Verification items for the finished model (mm, model axes). Face numbers are marked on the shaded views. A direction names the side the tool comes from. Give positions to 0.01 mm unless a question says otherwise; leave off trailing zeros. Write each loop counter-clockwise with the first axis right and the second up, starting at its lowest first coordinate (ties: lowest second). Pieces come first, ordered by that corner, then holes. Notation, with made-up numbers: (-11, 75.5) -> (18, 75.5) arc R11 cw to (18, 92.5) -> close; hole circle Ø3 at (8.25, -40). An arc over 180 degrees is marked (long way). Write item = value, one per line.
from build123d import *

# Parameters (mm, degrees)
F0_W      = 31.75
F0_H      = 31.75
F1_DEPTH  = 3.175
F3_D      = 2.54
F3_DEPTH  = 1.27
F3_TIP    = 0.7630929862
F4_W      = 31.75
F4_H      = 5.1026814207
F5_DEPTH  = 38.1
F6_W      = 21.6686837375
F6_H      = 5.1026814207
F7_DEPTH  = 19.05
F8_W      = 11.3971428946
F8_H      = 5.1026814207
F9_DEPTH  = 12.7
F10_W     = 5.5938977748
F10_H     = 5.1191067934
F11_DEPTH = 5.08
F12_SIZE  = 2.54
F14_ANGLE = -90
F15_R     = 1.5379719929
F16_DEPTH = 1.905


with BuildPart() as f1:
    # F0 (on Top) → F1 (new body)
    with BuildSketch(Plane.XY):
        Rectangle(F0_W, F0_H)
    extrude(amount=F1_DEPTH)

    # F3
    with Locations(Plane.XY.offset(3.175)):
        with Locations((-2.5495558511, 2.3657830898)):
            Hole(F3_D / 2, depth=F3_DEPTH)
            with Locations((0, 0, -(F3_DEPTH + F3_TIP / 2))):  # 118° drill point
                Cone(0, F3_D / 2, F3_TIP, mode=Mode.SUBTRACT)

    # F4 (on face) → F5 (join)
    with BuildSketch(Plane.XY.offset(3.175)):
        with Locations((0, 13.3236592896)):
            Rectangle(F4_W, F4_H)
    extrude(amount=F5_DEPTH)

    # F6 (on face) → F7 (join)
    with BuildSketch(Plane.XY.offset(41.275)):
        with Locations((0, 13.3236592896)):
            Rectangle(F6_W, F6_H)
    extrude(amount=F7_DEPTH)

    # F8 (on face) → F9 (join)
    with BuildSketch(Plane.XY.offset(60.325)):
        with Locations((0, 13.3236592896)):
            Rectangle(F8_W, F8_H)
    extrude(amount=F9_DEPTH)

    # F10 (on face) → F11 (join)
    with BuildSketch(Plane.XZ.offset(-10.7723185793)):
        with Locations((0, 70.4654466033)):
            Rectangle(F10_W, F10_H)
    extrude(amount=F11_DEPTH)

    # F12
    f12_edges = [f1.edges().sort_by_distance(p)[0] for p in [
        (0, 5.692319, 67.905893),
    ]]
    chamfer(f12_edges, length=F12_SIZE)


with BuildPart() as f1_1:
    # F14: moved
    add(f1.part.rotate(Axis((0, 15.8751159906, 0), (1, 0, 0)), F14_ANGLE))

    # F15 (on face) → F16 (join)
    with BuildSketch(Plane(origin=(0, 38.0691058929, -38.0691058929), x_dir=(1, 0, 0), z_dir=(0, -0.7071067812, 0.7071067812))):
        with Locations((0, 66.584341228)):
            Circle(F15_R)
    extrude(amount=F16_DEPTH)


solid = f1_1.part
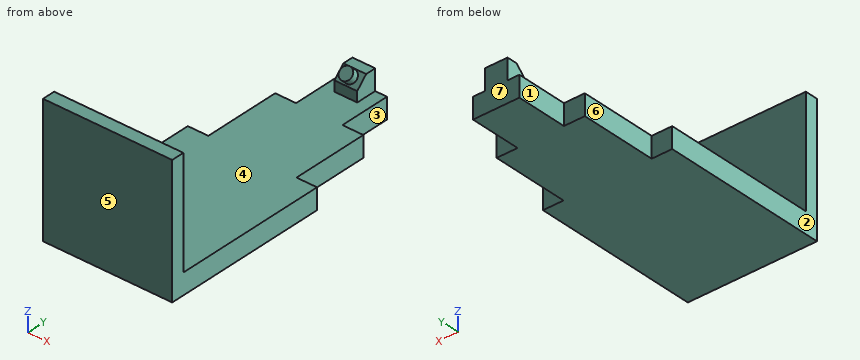
Item 1: Go/stop test with flat-tipped pins: P1, Ø4, axis at x = 4.5, y = 35, coming from the +Z side; P2, Ø4, axis at y = 64, z = 3, coming from the +X side; P3, Ø4, axis at x = -12, z = 9, coming from the +Y side; P4, Ø2, axis at y = 48.5, z = 7.5, coming from the +X side. Record where each tip stops, or that it passes through.
Response values:
P1 = 5.1
P2 = 10.83
P3 = 19.05
P4 = through
Item 2: Material ranges on line 1 (Y direction, x = 2, z = 7); line 2 (Y direction, x = -6.5, z = 25.5); line 3 (Z direction, x = -13.5, y = 32), recorded low to high.
Response values:
line_1 = 15.88 to 19.05, 83.78 to 88.9
line_2 = 15.88 to 19.05
line_3 = 0 to 5.1
Item 3: Sectioned sample at A-A on x = 4.5. Record the cut outline in (y, z), then the cut area to 3 significant figures.
Response values:
outline = (15.88, 0) -> (88.9, 0) -> (88.9, 5.1) -> (19.05, 5.1) -> (19.05, 31.75) -> (15.88, 31.75) -> close
area = 457 mm^2
Item 4: Mould release check, pull along Y, two halves, no side actions. Record for the marked faces 4, 5, 6 and 7: +Y half, -Y half, draft (parallel to the pull), parting line (faces both ways), or undercut.
Response values:
face_4 = undercut
face_5 = -Y half
face_6 = draft
face_7 = +Y half
Item 5: Sectioned sample at C-C on z = 19. Record the cut outline in (x, y) (3 decimals).
Response values:
outline = (-15.875, 15.875) -> (15.875, 15.875) -> (15.875, 19.05) -> (-15.875, 19.05) -> close
Item 6: Sectioned sample at B-B on y = 37. Record the cut outline in (x, z) (3 decimals), then the cut area to 3 significant figures.
Response values:
outline = (-15.875, 0) -> (15.875, 0) -> (15.875, 5.103) -> (-15.875, 5.103) -> close
area = 162 mm^2
Item 7: Sectioned sample at D-D on x = -13. Record the cut outline in (y, z), then the cut area to 3 significant figures.
Response values:
outline = (15.88, 0) -> (57.15, 0) -> (57.15, 5.1) -> (19.05, 5.1) -> (19.05, 31.75) -> (15.88, 31.75) -> close
area = 295 mm^2
Item 8: Set-up check for the marked faces 1, 2 and 3: record each of +Z, -Z, +X, -X, +Y, -Y from which the full face is reachable in a straight line by a thin tool's end or side.
Response values:
face_1 = +Z, -Z, -X, +Y
face_2 = +Z, -Z, -X, +Y, -Y
face_3 = +Z, -Z, +X, +Y
